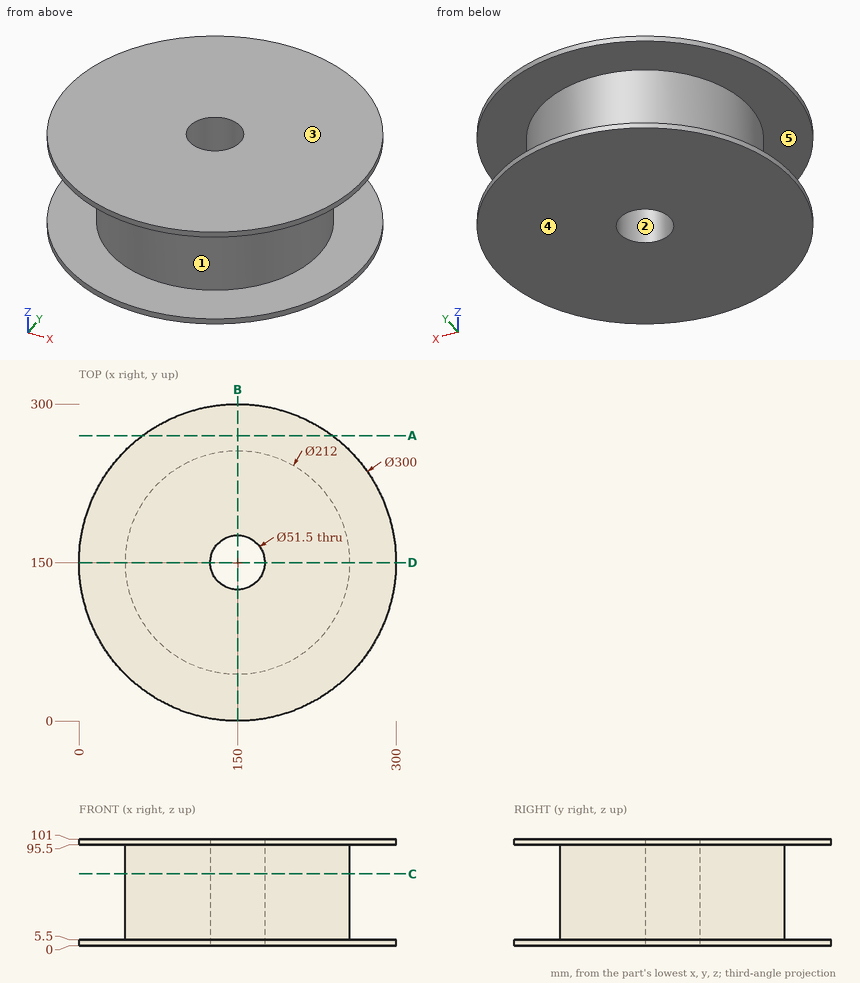
Check sheet for the drawn part. Datum: minimum x, y, z corner. Units: mm. A direction names the side the tool comes from. Give positions to 0.01 mm unless a question says otherwise; leave off trailing zeros. Order: outer loops, then holes, each group sorted by start corner. A loop starts at its lowest first (then second) coordinate and runs counter-clockwise, first axis right, second up. Notation, with made-up numbers: (38, -23.75) -> (59, -23.75) arc R13 cw to (59, 1.25) -> close; hole circle Ø1 at (68, 4). An arc over 180 degrees is marked (long way). One line per item, written item: value.
(1) Scan lines: line 1 along Z through (x, y) = (199, 288.5); line 2 along X through (y, z) = (150, 29); line 3 along Y through (x, z) = (128.5, 84). Record each from-to range of solid material in increasing order. Write a range as [from, to].
Final values:
line 1: [0, 5.5], [95.5, 101]
line 2: [44, 124.25], [175.75, 256]
line 3: [46.2, 135.83], [164.17, 253.8]
(2) Draft check along Z on the marked faces 3, 4 and 5. Enter one of: pulls with the +Z half, pulls with the -Z half, needs draft (parallel to the pull), parting line crosses it, or undercut.
Final values:
face 3: pulls with the +Z half
face 4: pulls with the -Z half
face 5: undercut
(3) Sectioned sample at C-C on z = 68. Record the cut outline in (x, y), then the cut area to 3 significant figures.
Final values:
outline: circle Ø212 at (150, 150); hole circle Ø51.5 at (150, 150)
area: 33,200 mm^2
(4) Sectioned sample at B-B on x = 150. Record the cut outline in (y, z).
Final values:
outline: (0, 0) -> (124.25, 0) -> (124.25, 101) -> (0, 101) -> (0, 95.5) -> (44, 95.5) -> (44, 5.5) -> (0, 5.5) -> close; (175.75, 0) -> (300, 0) -> (300, 5.5) -> (256, 5.5) -> (256, 95.5) -> (300, 95.5) -> (300, 101) -> (175.75, 101) -> close
(5) Sectioned sample at A-A on y = 270. Record the cut outline in (x, z).
Final values:
outline: (60, 0) -> (240, 0) -> (240, 5.5) -> (60, 5.5) -> close; (60, 95.5) -> (240, 95.5) -> (240, 101) -> (60, 101) -> close
(6) Gauge pin test, flat ends, axial feed: pin 1 (10 mm diameter, centred on x = 133, z = 50.5, fed in from +Y); pin 2 (1 mm diameter, centred on y = 148, z = 85.5, fed in from -X); pin 3 (1 mm diameter, centred on y = 131, z = 76.5, fed in from -X). Record the tip position at first contact, or that the pin passes through.
Final values:
pin 1: y = 255.32
pin 2: x = 44.01
pin 3: x = 45.63
(7) Tool access check on the marked faces 1 and 2. Record the directions out of +Z, -Z, +X, -X, +Y, -Y that give a thin tool (end or side, any length) a straight path to the whole face; none if there is none.
Final values:
face 1: none
face 2: +Z, -Z
